```python
from build123d import *

# Parameters (mm, degrees)
SKETCH3_W          = 35
SKETCH3_H          = 1.5
CHAMFER1_SIZE      = 0.45
CUT_EXTRUDE1_DEPTH = 1.19


with BuildPart() as part:
    # Sketch3 → Revolve1 (revolve)
    with BuildSketch(Plane(origin=(0, 0, 0), x_dir=(0, 0, -1), z_dir=(1, 0, 0))):
        with Locations((0, 0.75)):
            Rectangle(SKETCH3_W, SKETCH3_H)
    revolve(axis=Axis((0, 0, -17.5), (0, 0, 1)))

    # Chamfer1
    chamfer1_edges = [part.edges().sort_by_distance(p)[0] for p in [
        (0, -1.5, -17.5),
    ]]
    chamfer(chamfer1_edges, length=CHAMFER1_SIZE)

    # Sketch6 → Revolve2 (revolve)
    with BuildSketch(Plane(origin=(0, 0, 0), x_dir=(0, 0, -1), z_dir=(1, 0, 0))):
        Polygon((-17.5, 3), (-17.3, 3), (-15.8, 1.5), (-15.8, 0), (-17.5, 0), align=None)
    revolve(axis=Axis((0, 0, -17.5), (0, 0, 1)))

    # Sketch8 → Cut-Extrude1 (cut)
    with BuildSketch(Plane.XY.offset(17.5)):
        Polygon((0, 1.154700538), (-1, 0.577350269), (-1, -0.577350269), (0, -1.154700538), (1, -0.577350269), (1, 0.577350269), align=None)
    extrude(amount=-CUT_EXTRUDE1_DEPTH, mode=Mode.SUBTRACT)

    # Cut-Extrude2 cone 1 section (through the dimple's axis) → Cut-Extrude2 (revolve, cut)
    with BuildSketch(Plane(origin=(0, 0, 17.5), x_dir=(0, -1, 0), z_dir=(1, 0, 0))):
        Polygon((0, 0), (1.154700538, 0), (0, 1.154700538), align=None)
    revolve(axis=Axis((0, 0, 17.5), (0, 0, -1)), mode=Mode.SUBTRACT)


solid = part.part
```
Model file for the job. Use its own axes, mm. A direction names the side the tool comes from. Coordinates: 2 decimals unless noted, no trailing zeros. Order: outer loops, then holes, each group sorted by start corner. A loop starts at its lowest first (then second) coordinate and runs counter-clockwise, first axis right, second up. Notation, with made-up numbers: (8, 29) -> (14, 29) arc R21 ccw to (14, 38) -> close; hole circle Ø2 at (64, -28). An arc over 180 degrees is marked (long way). Return JSON: item names as keys, results as strings.
Item 1: Slice it at B-B (z = 8.5). Write the cut outline in (x, y).
Model answer:
{"outline": "circle Ø3 at (0, 0)"}
Item 2: Slice it at A-A (y = 0). Write the cut outline in (x, z).
Model answer:
{"outline": "(-3, 17.3) -> (-1.5, 15.8) -> (-1.5, -17.05) -> (-1.05, -17.5) -> (1.05, -17.5) -> (1.5, -17.05) -> (1.5, 15.8) -> (3, 17.3) -> (3, 17.5) -> (1.15, 17.5) -> (1, 17.35) -> (1, 16.31) -> (-1, 16.31) -> (-1, 17.35) -> (-1.15, 17.5) -> (-3, 17.5) -> close"}
Item 3: 3-axis set-ups, long thin cutter, end or side, ignore diameter. For faces 4 (the face through (0, 0, 16.31)), 5 (the face through (1, -1, 17.5)): which of +Z, -Z, +X, -X, +Y, -Y reach the whole face in a straight line?
Model answer:
{"face 4": "+Z", "face 5": "+Z, +X, -X, +Y, -Y"}
Item 4: Pin check, flat tips, straight feed: P1, Ø1, axis at x = 0.5, z = -9, coming from the +Y side; P2, Ø2, axis at y = -2, z = 12.5, coming from the +X side; P3, Ø1.5, axis at x = 2, y = -2.5, coming from the -Z side. Stop position of each tip, or through.
Model answer:
{"P1": "stops at y = 1.5", "P2": "stops at x = 1.12", "P3": "stops at z = 16.75"}
Item 5: Wall check: line 1 along Y through (x, z) = (-0.95, -11); line 2 along X through (y, z) = (-0.05, 2); line 3 along Z through (x, y) = (0.35, 0.55). Give the ranges that are in metal, low to high. Write a range as from..to.
Model answer:
{"line 1": "y = -1.16..1.16", "line 2": "x = -1.5..1.5", "line 3": "z = -17.5..16.31"}
Item 6: Mould opens along X. For faces 1 (the face through (0, 0, -17.5)), 2 (the face through (-0.07, -1.5, -0.85)), 3 (the face through (0.49, -0.87, 16.91)) say: pulls with the +X half, pulls with the -X half, needs draft (parallel to the pull), parting line crosses it, or undercut.
Model answer:
{"face 1": "needs draft", "face 2": "parting line crosses it", "face 3": "undercut"}
